from build123d import *

# Parameters (mm, degrees)
SKETCH_1_R               = 12.91
EXTRUDE_1_DEPTH          = 2.52
EXTRUDE_2_DEPTH          = 1
CUT_EXTRUDE_1_DEPTH      = 4
CUT_EXTRUDE_2_DEPTH      = 4
PATTERN_CIRCULAR_1_COUNT = 24


with BuildPart() as part:
    # 草图1 → 凸台-拉伸1 (new body)
    with BuildSketch(Plane(origin=(0, 0, 0), x_dir=(1, 0, 0), z_dir=(0, 1, 0))):
        with Locations(Location((0, 0, 0), (0, 0, 270))):
            Circle(SKETCH_1_R)
    extrude(amount=EXTRUDE_1_DEPTH)

    # 草图2 → 凸台-拉伸2 (add)
    with BuildSketch(Plane(origin=(0, 2.52, 0), x_dir=(1, 0, 0), z_dir=(0, 1, 0))):
        with BuildLine():
            Line((-2.8, 3.045), (2.8, 3.045))
            ThreePointArc((2.8, 3.045), (4.136668345, 0), (2.8, -3.045))
            Line((2.8, -3.045), (-2.8, -3.045))
            ThreePointArc((-2.8, -3.045), (-4.136668345, 0), (-2.8, 3.045))
        make_face()
    extrude(amount=EXTRUDE_2_DEPTH)

    # 草图3 → 切除-拉伸1 (cut)
    with BuildSketch(Plane(origin=(0, 3.52, 0), x_dir=(1, 0, 0), z_dir=(0, 1, 0))):
        with BuildLine():
            Line((-1.8, -2.045), (1.8, -2.045))
            ThreePointArc((1.8, -2.045), (2.724339369, 0), (1.8, 2.045))
            Line((1.8, 2.045), (-1.8, 2.045))
            ThreePointArc((-1.8, 2.045), (-2.724339369, 0), (-1.8, -2.045))
        make_face()
    extrude(amount=-CUT_EXTRUDE_1_DEPTH, mode=Mode.SUBTRACT)

    # 草图4 → 切除-拉伸2 (cut)
    with BuildSketch(Plane(origin=(0, 2.52, 0), x_dir=(1, 0, 0), z_dir=(0, 1, 0))):
        with BuildLine():
            Line((-11.175157972, -0.72), (-8.175157972, -0.72))
            ThreePointArc((-8.175157972, -0.72), (-8.011307018, 0), (-8.175157972, 0.72))
            Line((-8.175157972, 0.72), (-11.175157972, 0.72))
            ThreePointArc((-11.175157972, 0.72), (-11.339008927, 0), (-11.175157972, -0.72))
        make_face()
    cut_extrude_2 = extrude(amount=-CUT_EXTRUDE_2_DEPTH, mode=Mode.SUBTRACT)

    # 阵列(圆周)1: 切除-拉伸2 ×24 about axis
    pattern_circular_1_axis = Axis((0, 0, 0), (0, 1, 0))
    for i in range(1, PATTERN_CIRCULAR_1_COUNT):
        add(cut_extrude_2.rotate(pattern_circular_1_axis, i * 360 / PATTERN_CIRCULAR_1_COUNT), mode=Mode.SUBTRACT)


solid = part.part
The model under review builds one solid part; all positions refer to its coordinate system, in mm. Give positions to 0.01 mm unless a question says otherwise; leave off trailing zeros. Order: outer loops, then holes, each group sorted by start corner. A loop starts at its lowest first (then second) coordinate and runs counter-clockwise, first axis right, second up. Notation, with made-up numbers: (55.25, 42.5) -> (67.25, 42.5) arc R12 cw to (67.25, 60.5) -> close; hole circle Ø7 at (82.5, -30). An arc over 180 degrees is marked (long way). Write item = value, one per line. Start each with the question number.
(1) Take a section at A-A (z = 0). Write out the cut boundary in (x, y), plus the area to 3 significant figures.
(2) For L1, parallel to Z at x = 6.5, y = 0.2; L2, parallel to X at y = 0.5, z = -6.25; L3, parallel to X at y = 1, z = 3.75, list the stretches that pass through material, from the lowest coordinate up. Write a range as from..to.
(3) For pin 1 Ø4 at (x, z) = (3.5, 4) entering from -Y; pin 2 Ø2 at (x, y) = (5, 1) entering from -Z; pin 3 Ø2 at (y, z) = (1, 10) entering from -X; pin 4 Ø2 at (y, z) = (1, 9.5) entering from +X, all flat-tipped, find the tip position at first contact; note any pin that passes through.
(4) Take a section at C-C (y = 3). Write out the cut boundary in (x, z) (3 decimals).
(5) Take a section at D-D (y = 1.4). State how many separate pieces and enclosed holes the cut face has, plus the area to 3 significant figures.
(6) Take a section at B-B (x = 0). Write out the cut boundary in (y, z) (3 decimals), plus the area to 3 significant figures.
Returned:
q1.outline = (-12.91, 0) -> (-11.34, 0) -> (-11.34, 2.52) -> (-12.91, 2.52) -> close; (-8.01, 0) -> (-2.72, 0) -> (-2.72, 3.52) -> (-4.14, 3.52) -> (-4.14, 2.52) -> (-8.01, 2.52) -> close; (2.72, 0) -> (8.01, 0) -> (8.01, 2.52) -> (4.14, 2.52) -> (4.14, 3.52) -> (2.72, 3.52) -> close; (11.34, 0) -> (12.91, 0) -> (12.91, 2.52) -> (11.34, 2.52) -> close
q1.area = 37.4 mm²
q2.L1 = -11.15..-7.52, -5.48..5.48, 7.52..11.15
q2.L2 = -11.3..-7.27, -5.29..5.29, 7.27..11.3
q2.L3 = -12.35..-7.94, -7.12..7.12, 7.94..12.35
q3.pin_1 = 0
q3.pin_2 = -12.27
q3.pin_3 = -9.26
q3.pin_4 = 9.72
q4.outline = (-2.8, -3.045) -> (2.8, -3.045) arc R4.137 ccw to (2.8, 3.045) -> (-2.8, 3.045) arc R4.137 ccw to start; hole (-1.8, -2.045) -> (1.8, -2.045) arc R2.724 ccw to (1.8, 2.045) -> (-1.8, 2.045) arc R2.724 ccw to start
q5.separate_pieces = 1
q5.enclosed_holes = 25
q5.area = 392 mm²
q6.outline = (0, -12.91) -> (2.52, -12.91) -> (2.52, -11.339) -> (0, -11.339) -> close; (0, -8.011) -> (2.52, -8.011) -> (2.52, -3.045) -> (3.52, -3.045) -> (3.52, -2.045) -> (0, -2.045) -> close; (0, 2.045) -> (3.52, 2.045) -> (3.52, 3.045) -> (2.52, 3.045) -> (2.52, 8.011) -> (0, 8.011) -> close; (0, 11.339) -> (2.52, 11.339) -> (2.52, 12.91) -> (0, 12.91) -> close
q6.area = 40.0 mm²
